from build123d import *

# Parameters (mm, degrees)
F0_R     = 6
F1_DEPTH = 3


with BuildPart() as f1:
    # F0 (on Front) → F1 (new body)
    with BuildSketch(Plane.XZ):
        Polygon((-30, 65), (-40, 65), (-43, 65), (-43, 40), (-40, 40), (-40, 15), (-43, 15), (-43, 0), (-43, -15), (-40, -15), (-40, -40), (-43, -40), (-43, -65), (-40, -65), (-30, -65), (-30, -68), (-10, -68), (-10, -65), (0, -65), (10, -65), (10, -68), (30, -68), (30, -65), (40, -65), (43, -65), (43, -40), (40, -40), (40, -15), (43, -15), (43, 0), (43, 15), (40, 15), (40, 40), (43, 40), (43, 65), (40, 65), (30, 65), (30, 68), (10, 68), (10, 65), (0, 65), (-10, 65), (-10, 68), (-30, 68), align=None)
        with Locations((0, -25)):
            Circle(F0_R, mode=Mode.SUBTRACT)
    extrude(amount=F1_DEPTH)


solid = f1.part
Part model, mm, in its own coordinate system. A direction names the side the tool comes from. Coordinates: 2 decimals unless noted, no trailing zeros. Order: outer loops, then holes, each group sorted by start corner. A loop starts at its lowest first (then second) coordinate and runs counter-clockwise, first axis right, second up.
(1) Pull direction Z, two halves, no side cores. Call faces 5 (the face through (-37, -1, -65)), 6 (the face through (-41, -1, -40)), 7 (the face through (-1, -3, 1)): pulls with the +Z half, pulls with the -Z half, needs draft (parallel to the pull), parting line crosses it, or undercut.
Check sheet entries:
face 5: pulls with the -Z half
face 6: undercut
face 7: needs draft
(2) Slice it at C-C, the plane x = -32.5. Write the cut outline in (y, z), and give its area (3 significant figures).
Check sheet entries:
outline: (-3, -65) - (0, -65) - (0, 65) - (-3, 65) - close
area: 390 mm2
(3) Slice it at B-B, the plane z = -25. Write the cut outline in (x, y), and give its area (3 significant figures).
Check sheet entries:
outline: (-40, -3) - (-6, -3) - (-6, 0) - (-40, 0) - close; (6, -3) - (40, -3) - (40, 0) - (6, 0) - close
area: 204 mm2
(4) Tool access for faces 1 (the face through (-40, -1, 28)), 2 (the face through (-10, -1, 66)), 3 (the face through (-10, -1, -67)), 4 (the face through (42, -1, -40)): list every direction of +Z, -Z, +X, -X, +Y, -Y with a clear straight run to the whole face (end or side of a thin tool).
Check sheet entries:
face 1: -X, +Y, -Y
face 2: +Z, +Y, -Y
face 3: -Z, +Y, -Y
face 4: +X, +Y, -Y
(5) Pin check, flat tips, straight feed: pin 1 Ø1.5 at (y, z) = (-2, -66.5) entering from -X; pin 2 Ø1.5 at (x, y) = (36, -1) entering from +Z; pin 3 Ø1.5 at (y, z) = (-2, -67) entering from +X. Stop position of each tip, or through.
Check sheet entries:
pin 1: stops at x = -30
pin 2: stops at z = 65
pin 3: stops at x = 30
(6) Slice it at A-A, the plane x = 0. Write the cut outline in (y, z), and give its area (3 significant figures).
Check sheet entries:
outline: (-3, -65) - (0, -65) - (0, -31) - (-3, -31) - close; (-3, -19) - (0, -19) - (0, 65) - (-3, 65) - close
area: 354 mm2
(7) Probe L1, parallel to Z at x = 0, y = -1.9; L2, parallel to Z at x = 7, y = -0.55; L3, parallel to X at y = -0.9, z = 28.5. List the from-to ranges inside material, lowest first.
Check sheet entries:
L1: z = -65 to -31, -19 to 65
L2: z = -65 to 65
L3: x = -40 to 40
